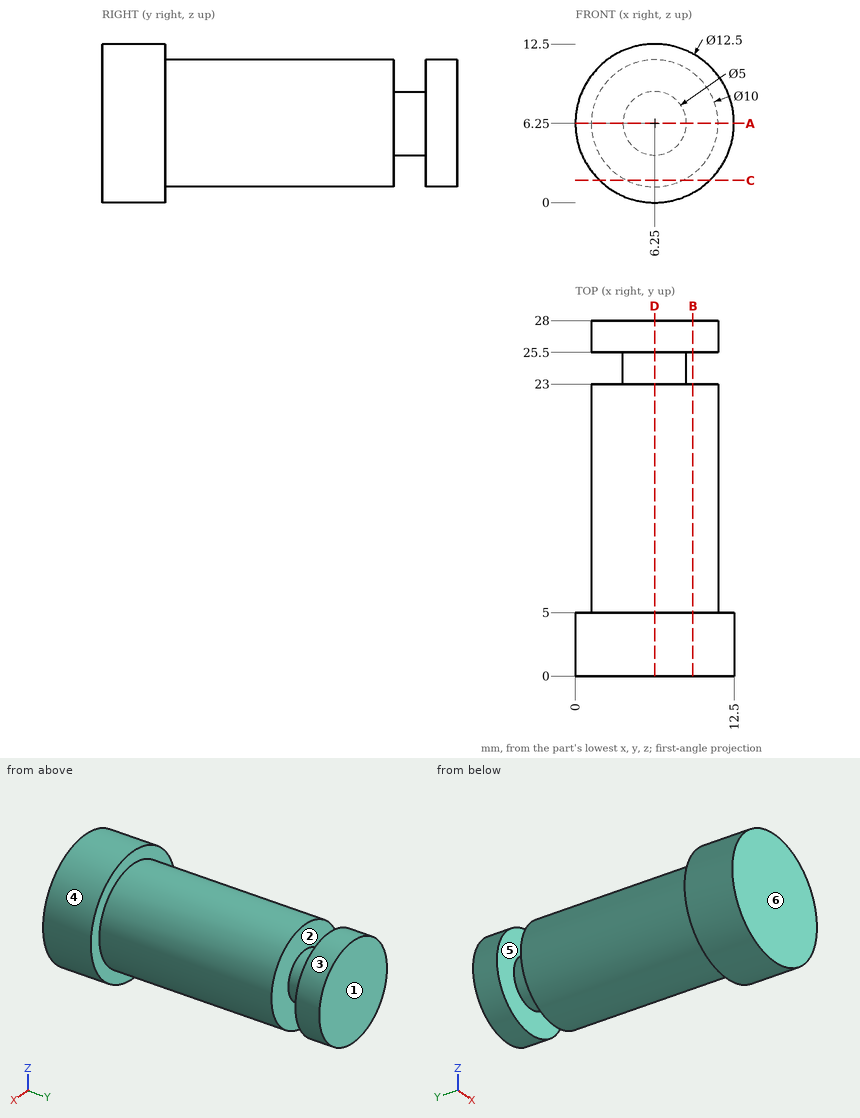
Geometry check sheet. Reference: drawing and pictorial views, mm from the part's lowest x, y, z. A direction names the side the tool comes from. Coordinates: 2 decimals unless noted, no trailing zeros. Order: outer loops, then holes, each group sorted by start corner. A loop starts at its lowest first (then second) coordinate and runs counter-clockwise, first axis right, second up.
Item 1: Scan lines: line 1 along Y through (x, z) = (10, 9); line 2 along Y through (x, z) = (3.25, 1.75); line 3 along Z through (x, y) = (6.25, 22.25). Record each from-to range of solid material in increasing order.
Item 2: Tool access check on the marked faces 1, 2 and 3. Record the directions out of +Z, -Z, +X, -X, +Y, -Y that give a thin tool (end or side, any length) a straight path to the whole face; none if there is none.
Item 3: Depth check by flat-ended pin: pin 1 (3 mm diameter, centred on y = 7, z = 3.5, fed in from +X); pin 2 (3 mm diameter, centred on y = 8.5, z = 2, fed in from +X); pin 3 (4 mm diameter, centred on x = 8.5, y = 13, fed in from -Z). Enter the tip coordinate at first touch or a pass-through.
Item 4: Mould release check, pull along Y, two halves, no side actions. Record for the marked faces 4, 5 and 6: released by +Y, released by -Y, zero draft, split by the parting line, or undercut.
Item 5: Section check A-A (z = 6.25). Enter the section's corners in (x, y).
Item 6: Section check D-D (x = 6.25). Enter the section's corners in (y, z).
Item 7: Section check B-B (x = 9.25). Enter the section's corners in (y, z).
Item 8: Section check C-C (z = 1.75). Enter the section's corners in (x, y).
Check sheet entries:
1. line 1: y = 0 to 23, 25.5 to 28
1. line 2: y = 0 to 5
1. line 3: z = 1.25 to 11.25
2. face 1: +Z, -Z, +X, -X, +Y
2. face 2: none
2. face 3: +Y
3. pin 1: stops at x = 11.09
3. pin 2: stops at x = 10.43
3. pin 3: stops at z = 1.26
4. face 4: zero draft
4. face 5: undercut
4. face 6: released by -Y
5. outline: (0, 0) - (12.5, 0) - (12.5, 5) - (11.25, 5) - (11.25, 23) - (8.75, 23) - (8.75, 25.5) - (11.25, 25.5) - (11.25, 28) - (1.25, 28) - (1.25, 25.5) - (3.75, 25.5) - (3.75, 23) - (1.25, 23) - (1.25, 5) - (0, 5) - close
6. outline: (0, 0) - (5, 0) - (5, 1.25) - (23, 1.25) - (23, 3.75) - (25.5, 3.75) - (25.5, 1.25) - (28, 1.25) - (28, 11.25) - (25.5, 11.25) - (25.5, 8.75) - (23, 8.75) - (23, 11.25) - (5, 11.25) - (5, 12.5) - (0, 12.5) - close
7. outline: (0, 0.77) - (5, 0.77) - (5, 2.25) - (23, 2.25) - (23, 10.25) - (5, 10.25) - (5, 11.73) - (0, 11.73) - close; (25.5, 2.25) - (28, 2.25) - (28, 10.25) - (25.5, 10.25) - close
8. outline: (1.91, 0) - (10.59, 0) - (10.59, 5) - (8.43, 5) - (8.43, 23) - (4.07, 23) - (4.07, 5) - (1.91, 5) - close; (4.07, 25.5) - (8.43, 25.5) - (8.43, 28) - (4.07, 28) - close
